from build123d import *

# Parameters (mm, degrees)
SKETCH_1_R          = 1.5
EXTRUDE_1_DEPTH     = 6
CHAMFER_1_SIZE      = 0.5
CUT_EXTRUDE_1_DEPTH = 10
CHAMFER_2_SIZE      = 0.5


with BuildPart() as part:
    # 草图1 → 凸台-拉伸1 (new body)
    with BuildSketch(Plane.XY):
        with BuildLine():
            Line((40.5, 11.25), (40.5, 12))
            Line((40.5, 12), (47, 12))
            Line((47, 12), (47, 0))
            Line((47, 0), (40.5, 0))
            Line((40.5, 0), (40.5, 0.75))
            ThreePointArc((40.5, 0.75), (40.060660172, 1.810660172), (39, 2.25))
            Line((39, 2.25), (8, 2.25))
            ThreePointArc((8, 2.25), (6.939339828, 1.810660172), (6.5, 0.75))
            Line((6.5, 0.75), (6.5, 0))
            Line((6.5, 0), (0, 0))
            Line((0, 0), (0, 12))
            Line((0, 12), (6.5, 12))
            Line((6.5, 12), (6.5, 11.25))
            ThreePointArc((6.5, 11.25), (6.939339828, 10.189339828), (8, 9.75))
            Line((8, 9.75), (39, 9.75))
            ThreePointArc((39, 9.75), (40.060660172, 10.189339828), (40.5, 11.25))
        make_face()
        with Locations((3.5, 3)):
            Circle(SKETCH_1_R, mode=Mode.SUBTRACT)
        with Locations((3.5, 9)):
            Circle(SKETCH_1_R, mode=Mode.SUBTRACT)
        with Locations((43.5, 3)):
            Circle(SKETCH_1_R, mode=Mode.SUBTRACT)
        with Locations((43.5, 9)):
            Circle(SKETCH_1_R, mode=Mode.SUBTRACT)
    extrude(amount=EXTRUDE_1_DEPTH)

    # 倒角1
    chamfer_1_edges = [part.edges().sort_by_distance(p)[0] for p in [
        (0, 12, 3),
        (47, 12, 3),
        (47, 0, 3),
        (0, 0, 3),
    ]]
    chamfer(chamfer_1_edges, length=CHAMFER_1_SIZE)

    # 草图2 → 切除-拉伸1 (cut)
    with BuildSketch(Plane(origin=(0, 9.75, 0), x_dir=(1, 0, 0), z_dir=(0, 1, 0))):
        with BuildLine():
            Line((30.829472469, -2), (15.737628945, -2))
            ThreePointArc((15.737628945, -2), (10.633550707, -3), (15.737628945, -4))
            Line((15.737628945, -4), (30.829472469, -4))
            ThreePointArc((30.829472469, -4), (35.933550707, -3), (30.829472469, -2))
        make_face()
    extrude(amount=-CUT_EXTRUDE_1_DEPTH, mode=Mode.SUBTRACT)

    # 倒角2
    chamfer_2_edges = [part.edges().sort_by_distance(p)[0] for p in [
        (2, 3, 0),
        (2, 3, 6),
        (2, 9, 0),
        (2, 9, 6),
        (42, 3, 0),
        (42, 3, 6),
        (42, 9, 0),
        (42, 9, 6),
    ]]
    chamfer(chamfer_2_edges, length=CHAMFER_2_SIZE)


solid = part.part
Can you work these out from the model? Positions are in its coordinate system, mm. A direction names the side the tool comes from. Coordinates: 2 decimals unless noted, no trailing zeros. Write each loop counter-clockwise with the first axis right and the second up, starting at its lowest first coordinate (ties: lowest second). Pieces come first, ordered by that corner, then holes.
Q1. Imagine slicing it at A-A, the plane z = 3. List the corners of the cut face in (x, y) for me.
Results found:
outline: (0, 0.5) - (0.5, 0) - (6.5, 0) - (6.5, 0.75) arc R1.5 cw to (8, 2.25) - (10.63, 2.25) - (10.63, 9.75) - (8, 9.75) arc R1.5 cw to (6.5, 11.25) - (6.5, 12) - (0.5, 12) - (0, 11.5) - close; (35.93, 2.25) - (39, 2.25) arc R1.5 cw to (40.5, 0.75) - (40.5, 0) - (46.5, 0) - (47, 0.5) - (47, 11.5) - (46.5, 12) - (40.5, 12) - (40.5, 11.25) arc R1.5 cw to (39, 9.75) - (35.93, 9.75) - close; hole circle Ø3 at (3.5, 3); hole circle Ø3 at (3.5, 9); hole circle Ø3 at (43.5, 3); hole circle Ø3 at (43.5, 9)
Q2. If we mould it in two halves opening along Y, with no side actions, what happens to faces 6 (the face through (3, 12, 3)), 7 (the face through (10.636, 6.052, 2.898)), 8 (the face through (4.19, 7.67, 2.96))? For each: +Y half, -Y half, draft (parallel to the pull), parting line (faces both ways), or undercut.
Results found:
face 6: +Y half
face 7: draft
face 8: undercut
Q3. Please list where these lines run through material, in increasing order: L1, parallel to Y at x = 43.5, z = 1.6; L2, parallel to X at y = 2, z = 1.7; L3, parallel to X at y = 4.25, z = 5.
Results found:
L1: y = 0 to 1.5, 4.5 to 7.5, 10.5 to 12
L2: x = 0 to 2.38, 4.62 to 7.17, 39.83 to 42.38, 44.62 to 47
L3: x = 0 to 2.67, 4.33 to 11.55, 15.02 to 31.55, 35.02 to 42.67, 44.33 to 47
Q4. For P1, Ø3, axis at x = 17.5, z = 3, coming from the -Y side; P2, Ø3.5, axis at x = 3.5, y = 3, coming from the -Z side; P3, Ø3, axis at x = 20.5, z = 2, coming from the +Y side, each with a flat end and sliding along its axis, tell me the tip position at first contact or that it passes through.
Results found:
P1: stops at y = 2.25
P2: stops at z = 0.25
P3: stops at y = 9.75
Q5. Imagine slicing it at C-C, the plane x = 29. List the corners of the cut face in (y, z) for me, plus the area to 3 significant figures.
Results found:
outline: (2.25, 0) - (9.75, 0) - (9.75, 2) - (2.25, 2) - close; (2.25, 4) - (9.75, 4) - (9.75, 6) - (2.25, 6) - close
area: 30.0 mm2
Q6. Which directions (+Z, -Z, +X, -X, +Y, -Y) give clear straight access to the entire face, cutting with the end or side of a thin tool? Please do faces 1 (the face through (40.07, 1.8, 2.96)), 2 (the face through (0, 6, 3)), 3 (the face through (6.93, 10.2, 2.96)), 4 (the face through (23, 6, 4)), 5 (the face through (43, 12, 3)).
Results found:
face 1: +Z, -Z, -Y
face 2: +Z, -Z, -X, +Y, -Y
face 3: +Z, -Z, +Y
face 4: +Y, -Y
face 5: +Z, -Z, +X, -X, +Y
Q7. Imagine slicing it at D-D, the plane x = 3.5. List the corners of the cut face in (y, z) for me, plus the area to 3 significant figures.
Results found:
outline: (0, 0) - (1, 0) - (1.5, 0.5) - (1.5, 5.5) - (1, 6) - (0, 6) - close; (4.5, 0.5) - (5, 0) - (7, 0) - (7.5, 0.5) - (7.5, 5.5) - (7, 6) - (5, 6) - (4.5, 5.5) - close; (10.5, 0.5) - (11, 0) - (12, 0) - (12, 6) - (11, 6) - (10.5, 5.5) - close
area: 35.0 mm2
Q8. Imagine slicing it at B-B, the plane y = 9. List the corners of the cut face in (x, z) for me, plus the area to 3 significant figures.
Results found:
outline: (0, 0) - (1.5, 0) - (2, 0.5) - (2, 5.5) - (1.5, 6) - (0, 6) - close; (5, 0.5) - (5.5, 0) - (41.5, 0) - (42, 0.5) - (42, 5.5) - (41.5, 6) - (5.5, 6) - (5, 5.5) - close; (45, 0.5) - (45.5, 0) - (47, 0) - (47, 6) - (45.5, 6) - (45, 5.5) - close; hole (15.74, 2) - (30.83, 2) arc R2.65 ccw (long way) to (30.83, 4) - (15.74, 4) arc R2.65 ccw (long way) to start
area: 171 mm2
